Can you work these out from the model? Positions are in its coordinate system, mm. A direction names the side the tool comes from. Coordinates: 2 decimals unless noted, no trailing zeros. Loops run counter-clockwise (first coordinate to the right, second up) from the corner with the lowest first, then second, coordinate; pieces in that order, holes last. Notation, with made-up numbers: (6.25, 2) -> (42.25, 2) arc R16 ccw to (42.25, 9) -> close; hole circle Ø7 at (-4.75, 86.25). An arc over 180 degrees is marked (long way). Use one line per item in the form item = value. Start each with the question number.
(1) Imagine slicing it at D-D (y = -37). List the corners of the cut face in (x, z) for me, plus the area to 3 significant figures.
(2) I'm going to push flat-ended pins straight in: pin 1 (10 mm diameter, centred on x = 19, y = 19, fed in from +Z); pin 2 (2 mm diameter, centred on y = 13.5, z = 1.5, fed in from +X); pin 3 (10 mm diameter, centred on x = 32, y = 25, fed in from +Z). Where does each tip first touch, or does it pass through?
(3) Imagine slicing it at B-B (z = 14). State how many separate pieces and enclosed holes the cut face has, plus the area to 3 significant figures.
(4) Thinking about a two-plate mould opening in Z: for faces 1 (the flat face through (55, 0, 9.5)), 2 (the flat face through (12, -37, 9)), 3 (the cylindrical face through (38.8, 14.25, 3.72)), 4 (the flat face through (-40, -37, 5.5)), which applies, released by +Z, released by -Z, zero draft, split by the parting line, or undercut?
(5) Imagine slicing it at A-A (y = 0). List the corners of the cut face in (x, z) for me.
(6) I need wall thicknesses on line 1 (Y direction, x = -44, z = 14.75); line 2 (X direction, y = 24, z = 2.5); line 3 (X direction, y = 17, z = 11.75). Which ranges of each line are inside material? Lowest first, please. Write a range as [from, to].
(7) On a 3-axis mill with a long thin cutter (end or side, diameter ignored), from which of +Z, -Z, +X, -X, +Y, -Y can I reach the whole of each face in a straight line? I mean faces 5 (the flat face through (-14, 19, 5.1)), 6 (the cylindrical face through (-9.5, 0.1, 0.9)), 7 (the flat face through (-20, 0, 0.6)), 8 (the flat face through (-40, -1, -6)). Say none if no direction works.
(8) Imagine slicing it at C-C (x = 44). List the corners of the cut face in (y, z) for me.
```python
from build123d import *

# Parameters (mm, degrees)
PAD_DEPTH       = 41
POCKET_DEPTH    = 33
POCKET001_DEPTH = 1.5
SKETCH007_R     = 4
SKETCH007_R_2   = 1.95
SKETCH007_R_3   = 2
PAD005_DEPTH    = 6
SKETCH008_W     = 14
SKETCH008_H     = 10
POCKET002_DEPTH = 40
SKETCH013_R     = 1.95
POCKET003_DEPTH = 8
SKETCH018_W     = 39.6
SKETCH018_H     = 12
SKETCH018_H_2   = 9
PAD012_DEPTH    = 17
SKETCH019_W     = 35.9
SKETCH019_H     = 56.1
POCKET006_DEPTH = 11.9
SKETCH023_W     = 79.5
SKETCH023_H     = 6
POCKET007_DEPTH = 0.6
SKETCH024_W     = 80
SKETCH024_H     = 0.5
PAD016_DEPTH    = 2
PAD017_DEPTH    = 10
SKETCH026_W     = 8
SKETCH026_H     = 16
POCKET008_DEPTH = 16


with BuildPart() as part:
    # Sketch → Pad (new body, symmetric)
    with BuildSketch(Plane.XZ):
        Polygon((-48, 17), (-48, -6), (-32, -6), (-32, 0), (48, 0), (48, 17), align=None)
    extrude(amount=PAD_DEPTH, both=True)

    # Sketch001 → Pocket (cut, symmetric)
    with BuildSketch(Plane.XZ):
        Polygon((-33, 1.5), (47, 1.5), (47, 18.5), (-47, 18.5), (-47, -4.5), (-33, -4.5), align=None)
    extrude(amount=POCKET_DEPTH, both=True, mode=Mode.SUBTRACT)

    # Sketch004 → Pocket001 (cut)
    with BuildSketch(Plane.XY):
        with BuildLine():
            ThreePointArc((-4.5, 5), (-9.5, 0), (-4.5, -5))
            Line((-4.5, -5), (20.5, -5))
            ThreePointArc((20.5, -5), (25.5, 0), (20.5, 5))
            Line((20.5, 5), (-4.5, 5))
        make_face()
    extrude(amount=POCKET001_DEPTH, mode=Mode.SUBTRACT)

    # Sketch007 → Pad005 (join)
    with BuildSketch(Plane.XY):
        with Locations((15, 15)):
            Circle(SKETCH007_R)
        with Locations((15, 15)):
            Circle(SKETCH007_R_2, mode=Mode.SUBTRACT)
        with Locations((37, 15)):
            Circle(SKETCH007_R)
        with Locations((37, 15)):
            Circle(SKETCH007_R_2, mode=Mode.SUBTRACT)
        with Locations((26, -16)):
            Circle(SKETCH007_R_3)
    extrude(amount=PAD005_DEPTH)

    # Sketch008 → Pocket002 (cut, symmetric)
    with BuildSketch(Plane.XZ):
        with Locations((-40, 0.5)):
            Rectangle(SKETCH008_W, SKETCH008_H)
    extrude(amount=POCKET002_DEPTH, both=True, mode=Mode.SUBTRACT)

    # Sketch013 (on DatumPlane) → Pocket003 (cut)
    with BuildSketch(Plane.XY.offset(17)):
        with Locations((-44, 37)):
            Circle(SKETCH013_R)
        with Locations((12, 37)):
            Circle(SKETCH013_R)
        with Locations((44, 37)):
            Circle(SKETCH013_R)
        with Locations((44, -37)):
            Circle(SKETCH013_R)
        with Locations((12, -37)):
            Circle(SKETCH013_R)
        with Locations((-44, -37)):
            Circle(SKETCH013_R)
    extrude(amount=-POCKET003_DEPTH, mode=Mode.SUBTRACT)

    # Sketch018 → Pad012 (join)
    with BuildSketch(Plane.XY):
        with Locations((-13.2, 19.8)):
            Rectangle(SKETCH018_W, SKETCH018_H)
        with Locations((-13.2, -28.5)):
            Rectangle(SKETCH018_W, SKETCH018_H_2)
    extrude(amount=PAD012_DEPTH)

    # Sketch019 (on DatumPlane) → Pocket006 (cut)
    with BuildSketch(Plane.XY.offset(17)):
        with Locations((-13.25, -4.95)):
            Rectangle(SKETCH019_W, SKETCH019_H)
    extrude(amount=-POCKET006_DEPTH, mode=Mode.SUBTRACT)

    # Sketch023 → Pocket007 (cut)
    with BuildSketch(Plane.XY):
        with Locations((7.75, 0)):
            Rectangle(SKETCH023_W, SKETCH023_H)
    extrude(amount=POCKET007_DEPTH, mode=Mode.SUBTRACT)

    # Sketch024 → Pad016 (join)
    with BuildSketch(Plane.XY):
        with Locations((8, 40.75)):
            Rectangle(SKETCH024_W, SKETCH024_H)
        with Locations((8, -40.75)):
            Rectangle(SKETCH024_W, SKETCH024_H)
    extrude(amount=-PAD016_DEPTH)

    # Sketch025 → Pad017 (join)
    with BuildSketch(Plane.XY):
        with BuildLine():
            Line((48, 13), (48, -13))
            ThreePointArc((52, -9), (49.171573, -10.171573), (48, -13))
            Line((64, -9), (52, -9))
            ThreePointArc((64, -9), (64.707107, -8.707107), (65, -8))
            Line((65, 8), (65, -8))
            ThreePointArc((65, 8), (64.707107, 8.707107), (64, 9))
            Line((52, 9), (64, 9))
            ThreePointArc((48, 13), (49.171573, 10.171573), (52, 9))
        make_face()
    extrude(amount=PAD017_DEPTH)

    # Sketch026 (on Face12 of Pad017) → Pocket008 (cut)
    with BuildSketch(Plane(origin=(47, 0, 0), x_dir=(0, 0, -1), z_dir=(-1, 0, 0))):
        with Locations((-5.5, 0)):
            Rectangle(SKETCH026_W, SKETCH026_H)
    extrude(amount=-POCKET008_DEPTH, mode=Mode.SUBTRACT)


solid = part.part
```
Worked out:
q1.outline = (-48, -6) -> (-32, -6) -> (-32, 0) -> (48, 0) -> (48, 17) -> (45.95, 17) -> (45.95, 9) -> (42.05, 9) -> (42.05, 17) -> (13.95, 17) -> (13.95, 9) -> (10.05, 9) -> (10.05, 17) -> (-42.05, 17) -> (-42.05, 9) -> (-45.95, 9) -> (-45.95, 17) -> (-48, 17) -> close; hole (-47, -4.5) -> (-33, -4.5) -> (-33, 5.5) -> (-47, 5.5) -> close
q1.area = 1,490 mm2
q2.pin_1 = 6
q2.pin_2 = 48.03
q2.pin_3 = 1.5
q3.separate_pieces = 2
q3.enclosed_holes = 7
q3.area = 1,770 mm2
q4.face_1 = undercut
q4.face_2 = released by +Z
q4.face_3 = zero draft
q4.face_4 = undercut
q5.outline = (-48, -6) -> (-32, -6) -> (-32, 0.6) -> (-9.5, 0.6) -> (-9.5, 1.5) -> (-33, 1.5) -> (-33, -4.5) -> (-47, -4.5) -> (-47, 17) -> (-48, 17) -> close; (25.5, 0.6) -> (47.5, 0.6) -> (47.5, 0) -> (65, 0) -> (65, 10) -> (48, 10) -> (48, 17) -> (47, 17) -> (47, 9.5) -> (63, 9.5) -> (63, 1.5) -> (25.5, 1.5) -> close
q6.line_1 = [-41, -38.95], [-35.05, -33], [33, 35.05], [38.95, 41]
q6.line_2 = [-48, -47], [-33, 6.6], [47, 48]
q6.line_3 = [-48, -47], [-33, -31.2], [4.7, 6.6], [47, 48]
q7.face_5 = +Z
q7.face_6 = +Z, -Z
q7.face_7 = -Z
q7.face_8 = -Z, +X, -X, +Y, -Y
q8.outline = (-41, -2) -> (-40.5, -2) -> (-40.5, 0) -> (-3, 0) -> (-3, 0.6) -> (3, 0.6) -> (3, 0) -> (40.5, 0) -> (40.5, -2) -> (41, -2) -> (41, 17) -> (38.95, 17) -> (38.95, 9) -> (35.05, 9) -> (35.05, 17) -> (33, 17) -> (33, 1.5) -> (-33, 1.5) -> (-33, 17) -> (-35.05, 17) -> (-35.05, 9) -> (-38.95, 9) -> (-38.95, 17) -> (-41, 17) -> close
